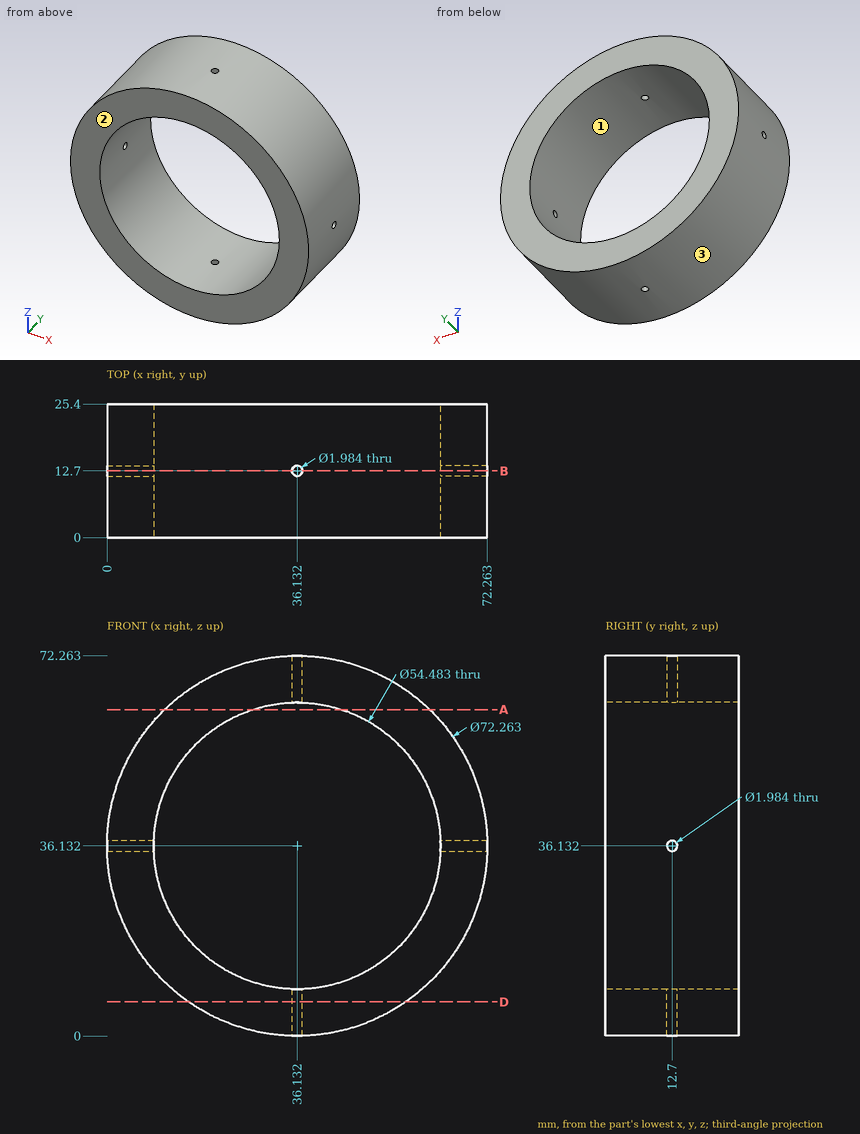
The figure shows three views and two pictorial views of one solid part (mm, origin at its lowest corner). Answer the questions. Coordinates: 2 decimals unless noted, no trailing zeros. Loops run counter-clockwise (first coordinate to the right, second up) from the corner with the lowest first, then second, coordinate; pieces in that order, holes last. Notation, with made-up numbers: (-24.75, 4.5) - (34.25, 4.5) arc R23 ccw to (34.25, 25.5) - close; hole circle Ø5 at (50.25, -16.5). An arc over 180 degrees is marked (long way). Use a Markdown table: item, result. Add a question column.
1) Find the intervals of material crossed by line 1 (Z direction, x = 55.5, y = 20.25) (1 decimal); line 2 (X direction, y = 13, z = 31) (1 decimal); line 3 (Z direction, x = 40.5, y = 16) (1 decimal), in increasing order.
2) The mould has two halves that part along Z. Classify the marked faces 1, 2 and 3: released by +Z, released by -Z, zero draft, split by the parting line, or undercut.
3) The part is cut by section D-D, the plane z = 6.5. Give the vertices of the cut face in (x, y) (1 decimal).
4) The part is cut by section B-B, the plane y = 12.7. State how many separate pieces and enclosed holes the cut face has, and give its area (3 significant figures).
5) Given pin 1 (2.5 mm diameter, centred on x = 36.13, y = 12.7, fed in from -Z); pin 2 (2 mm diameter, centred on x = 15.5, y = 20, fed in from -Z); pin 3 (5 mm diameter, centred on x = 52, y = 13.5, fed in from -Z) (1 decimal); pin 4 (3 mm diameter, centred on y = 19.5, z = 50.5, fed in from +X), each flat-ended and moving along its own axis, determine where each tip first touches the part or whether it passes through.
6) The part is cut by section A-A, the plane z = 62. Give the vertices of the cut face in (x, y).
Here are the results:
| question | item | result |
|---|---|---|
| 1 | line 1 | z = 5.6 to 17, 55.3 to 66.6 |
| 1 | line 2 | x = 0.4 to 9.4, 62.9 to 71.9 |
| 1 | line 3 | z = 0.3 to 9.2, 63 to 72 |
| 2 | face 1 | undercut |
| 2 | face 2 | zero draft |
| 2 | face 3 | split by the parting line |
| 3 | outline | (15.5, 0) - (56.8, 0) - (56.8, 25.4) - (15.5, 25.4) - close; hole circle Ø2 at (36.1, 12.7) |
| 4 | separate pieces | 4 |
| 4 | enclosed holes | 0 |
| 4 | area | 1,700 mm^2 |
| 5 | pin 1 | stops at z = 0 |
| 5 | pin 2 | stops at z = 5.8 |
| 5 | pin 3 | stops at z = 2.6 |
| 5 | pin 4 | stops at x = 69.89 |
| 6 | outline | (10.91, 0) - (27.59, 0) - (27.59, 25.4) - (10.91, 25.4) - close; (44.67, 0) - (61.36, 0) - (61.36, 25.4) - (44.67, 25.4) - close |
